Here's the drawing with two shaded views (mm, measured from the low corner). I have some questions. A direction names the side the tool comes from. Give positions to 0.01 mm unless a question says otherwise; leave off trailing zeros. Write each loop counter-clockwise with the first axis right and the second up, starting at its lowest first coordinate (ties: lowest second). Pieces come first, ordered by that corner, then holes. Notation, with made-up numbers: (-27, 82.5) -> (-18, 82.5) arc R33 cw to (-18, 110.5) -> close; hole circle Ø4 at (60.25, 62). An arc over 180 degrees is marked (long way). One line per question, with ' | ' between items.
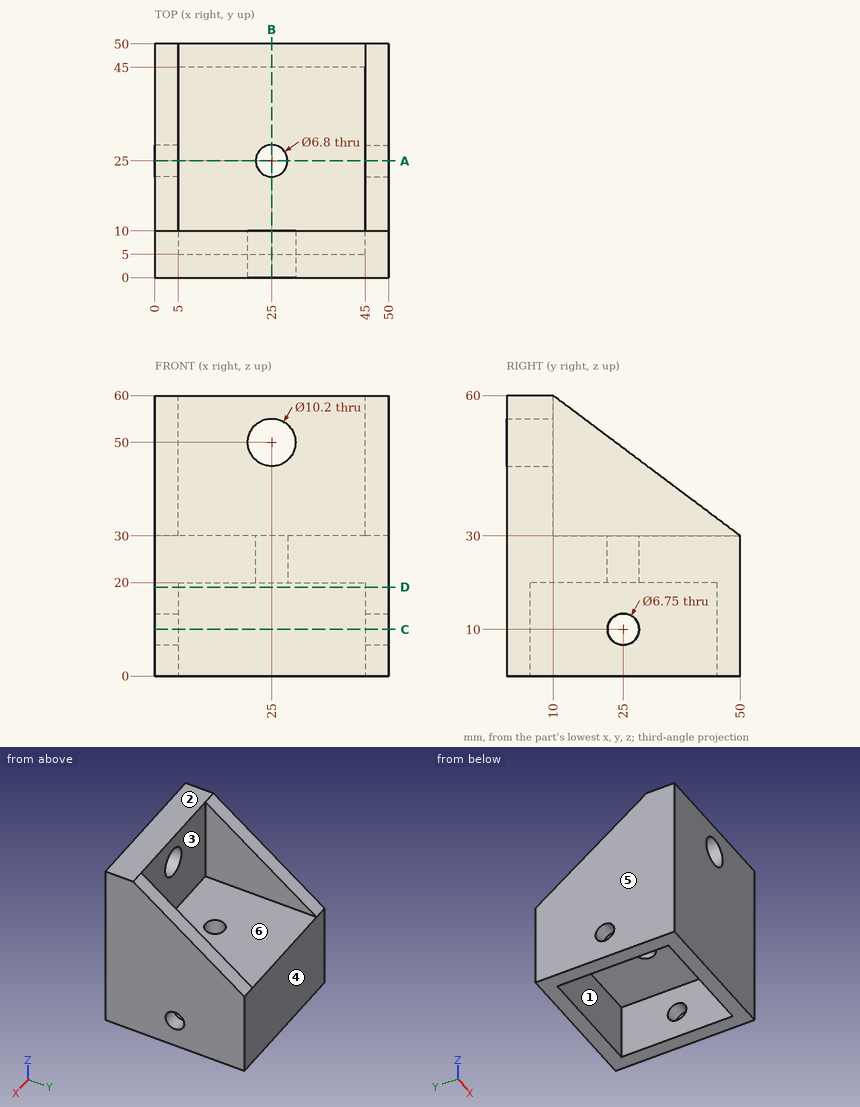
Q1. If I drill on line 1 along Y through (x, z) = (23.5, 16); line 2 along X through (y, z) = (7.5, 51), over which ranges is the centre line in solid material (lowest first)?
Answer below:
line 1: y = 0 to 5, 45 to 50 | line 2: x = 0 to 20, 30 to 50
Q2. Will these pins go through, and if not, where does the flat tip stop? pin 1 (3 mm diameter, centred on x = 23.5, z = 44, fed in from +Y); pin 2 (6 mm diameter, centred on x = 25, z = 50, fed in from +Y); pin 3 (1.5 mm diameter, centred on x = 32.5, y = 17.5, fed in from +Z); pin 4 (8 mm diameter, centred on x = 25, y = 25, fed in from -Z).
Answer below:
pin 1: stops at y = 10 | pin 2: passes through | pin 3: stops at z = 30 | pin 4: stops at z = 20
Q3. Imagine slicing it at C-C on z = 10. Please give me the cut outline in (x, y) (3 decimals), and give its area (4 significant figures).
Answer below:
outline: (0, 0) -> (50, 0) -> (50, 21.625) -> (45, 21.625) -> (45, 5) -> (5, 5) -> (5, 21.625) -> (0, 21.625) -> close; (0, 28.375) -> (5, 28.375) -> (5, 45) -> (45, 45) -> (45, 28.375) -> (50, 28.375) -> (50, 50) -> (0, 50) -> close | area: 832.5 mm^2
Q4. Imagine slicing it at D-D on z = 19. Please give me the cut outline in (x, y).
Answer below:
outline: (0, 0) -> (50, 0) -> (50, 50) -> (0, 50) -> close; hole (5, 5) -> (45, 5) -> (45, 45) -> (5, 45) -> close
Q5. Imagine slicing it at B-B on x = 25. Please give me the cut outline in (y, z).
Answer below:
outline: (0, 0) -> (5, 0) -> (5, 20) -> (21.6, 20) -> (21.6, 30) -> (10, 30) -> (10, 44.9) -> (0, 44.9) -> close; (0, 55.1) -> (10, 55.1) -> (10, 60) -> (0, 60) -> close; (28.4, 20) -> (45, 20) -> (45, 0) -> (50, 0) -> (50, 30) -> (28.4, 30) -> close
Q6. If we mould it in two halves opening along X, with no side actions, what happens to the marked faces 4, 5 and 6? For each: +X half, -X half, draft (parallel to the pull), parting line (faces both ways), or undercut.
Answer below:
face 4: draft | face 5: -X half | face 6: undercut
Q7. On a 3-axis mill with a long thin cutter (end or side, diameter ignored), from which of +Z, -Z, +X, -X, +Y, -Y can I reach the whole of each face in a straight line? I mean the marked faces 1, 2 and 3. Say none if no direction works.
Answer below:
face 1: -Z | face 2: +Z, +X, -X, +Y, -Y | face 3: +Z, +Y
Q8. Imagine slicing it at A-A on y = 25. Please give me the cut outline in (x, z) (3 decimals), and give its area (3 significant figures).
Answer below:
outline: (0, 0) -> (5, 0) -> (5, 6.625) -> (0, 6.625) -> close; (0, 13.375) -> (5, 13.375) -> (5, 20) -> (21.6, 20) -> (21.6, 30) -> (5, 30) -> (5, 48.75) -> (0, 48.75) -> close; (28.4, 20) -> (45, 20) -> (45, 13.375) -> (50, 13.375) -> (50, 48.75) -> (45, 48.75) -> (45, 30) -> (28.4, 30) -> close; (45, 0) -> (50, 0) -> (50, 6.625) -> (45, 6.625) -> close | area: 752 mm^2
